Autodesk Inventor part; units mm, degrees
ref_plane "YZ Plane" through (0, 0, 0) normal (1, 0, 0) x (0, 1, 0)
ref_plane "XZ Plane" through (0, 0, 0) normal (0, 1, 0) x (-1, 0, 0)
ref_plane "XY Plane" through (0, 0, 0) normal (0, 0, 1) x (1, 0, 0)
sketch "Sketch1" plane through (0, 0, 0) normal (0, 0, 1) x (1, 0, 0)
  line L0 (0, 0) -> (25.4, 0)
  line L1 (25.4, 0) -> (25.4, 50.8)
  line L2 (25.4, 50.8) -> (0, 50.8)
  line L3 (0, 50.8) -> (0, 0)
  dimension "d0" = 25.4
  dimension "d1" = 50.8
extrude "Extrusion1" add sketch "Sketch1" along normal blind 279.4
shell "Shell1" thickness 3.175 removed faces 2 at (8.4667, 33.8667, 0) at (8.4667, 33.8667, 279.4)
sketch "Sketch2" plane through (25.4, 0, 0) normal (1, 0, 0) x (0, 0, -1)
  line L0 (-279.4, 50.8) -> (-279.4, 0)
  line L1 (0, 50.8) -> (-279.4, 50.8)
  circle A0 centre (-266.7, 38.1) radius 2.3813
  dimension "d5" = 4.7625
  dimension "d6" = 12.7
  dimension "d7" = 12.7
extrude "Extrusion2" cut sketch "Sketch2" against normal through all
pattern_linear "Rectangular Pattern1" count 11 spacing 25.4 along (0, 0, -1) count 2 spacing 25.4 along (0, -1, 0) of "Extrusion2"
sketch "Sketch3" plane through (0, 50.8, 0) normal (0, 1, 0) x (1, 0, 0)
  line L0 (0, -279.4) -> (25.4, -279.4)
  line L1 (25.4, 0) -> (25.4, -279.4)
  line L2 (0, -279.4) -> (25.4, -279.4)
  line L3 (25.4, -228.6) -> (0, -279.4)
  dimension "d16" = 50.8
extrude "Extrusion3" cut sketch "Sketch3" against normal through all
properties part number "Frame_MidRollerSupport"
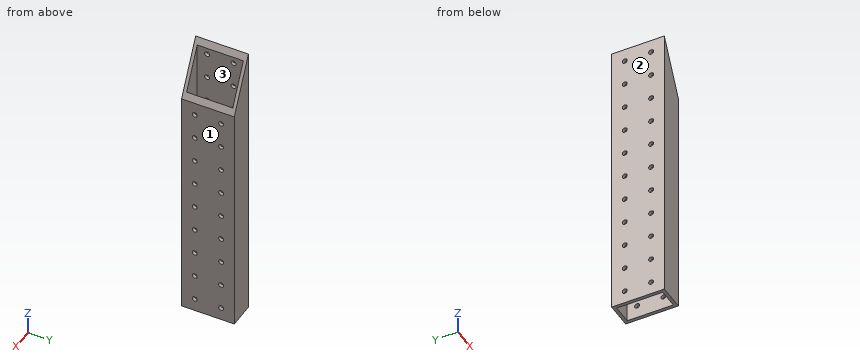
Can you work these out from the model? Positions are in its coordinate system, mm. Face numbers are marked on the shaded views. Give positions to 0.01 mm unless a question says otherwise; leave off trailing zeros. Order: outer loops, then holes, each group sorted by start corner. A loop starts at its lowest first (then second) coordinate and runs counter-clockwise, first axis right, second up. Notation, with made-up numbers: (15.25, 68.5) - (73.25, 68.5) arc R24 ccw to (73.25, 83.5) - close; hole circle Ø4 at (46.5, 51.25). An arc over 180 degrees is marked (long way). Use a Markdown table: item, result. Add a question column.
Q1. If we mould it in two halves opening along X, with no side actions, what happens to the marked faces 1, 2 and 3? For each: released by +X, released by -X, zero draft, split by the parting line, or undercut.
Q2. If we section it at A-A on z = 165.1: Write out the boundary of the cut face in (x, y) (3 decimals), plus the area to 3 significant figures.
Q3. Please list where these lines run through material, in increasing order: line 1 along Y through (x, z) = (23.7, 165.1); line 2 along Y through (x, z) = (9.75, 171.5) (3 decimals); line 3 along X through (y, z) = (40.5, 227.5) (3 decimals).
Q4. If we section it at D-D on z = 43: Write out the boundary of the cut face in (x, y) (3 decimals).
Q5. If we section it at C-C on z = 266.7: Write out the boundary of the cut face in (x, y) (3 decimals).
Q6. If we section it at B-B on y = 23: Write out the boundary of the cut face in (x, z) (3 decimals), plus the area to 3 significant figures.
Answers follow:
| question | item | result |
|---|---|---|
| 1 | face 1 | released by +X |
| 1 | face 2 | released by -X |
| 1 | face 3 | undercut |
| 2 | outline | (0, 0) - (25.4, 0) - (25.4, 10.319) - (22.225, 10.319) - (22.225, 3.175) - (3.175, 3.175) - (3.175, 10.319) - (0, 10.319) - close; (0, 15.081) - (3.175, 15.081) - (3.175, 35.719) - (0, 35.719) - close; (0, 40.481) - (3.175, 40.481) - (3.175, 47.625) - (22.225, 47.625) - (22.225, 40.481) - (25.4, 40.481) - (25.4, 50.8) - (0, 50.8) - close; (22.225, 15.081) - (25.4, 15.081) - (25.4, 35.719) - (22.225, 35.719) - close |
| 2 | area | 383 mm^2 |
| 3 | line 1 | y = 0 to 10.32, 15.08 to 35.72, 40.48 to 50.8 |
| 3 | line 2 | y = 0 to 3.175, 47.625 to 50.8 |
| 3 | line 3 | x = 0 to 3.175, 22.225 to 25.4 |
| 4 | outline | (0, 0) - (25.4, 0) - (25.4, 50.8) - (0, 50.8) - close; hole (3.175, 3.175) - (22.225, 3.175) - (22.225, 47.625) - (3.175, 47.625) - close |
| 5 | outline | (0, 0) - (6.35, 0) - (6.35, 3.175) - (3.175, 3.175) - (3.175, 10.319) - (0, 10.319) - close; (0, 15.081) - (3.175, 15.081) - (3.175, 35.719) - (0, 35.719) - close; (0, 40.481) - (3.175, 40.481) - (3.175, 47.625) - (6.35, 47.625) - (6.35, 50.8) - (0, 50.8) - close |
| 6 | outline | (0, 0) - (3.175, 0) - (3.175, 273.05) - (0, 279.4) - close; (22.225, 0) - (25.4, 0) - (25.4, 228.6) - (22.225, 234.95) - close |
| 6 | area | 1,610 mm^2 |
